The listing builds one solid part. Answer for the finished solid, in the listing's coordinates (mm). Give positions to 0.01 mm unless a question says otherwise; leave off trailing zeros. Order: outer loops, then holes, each group sorted by start corner. A loop starts at its lowest first (then second) coordinate and runs counter-clockwise, first axis right, second up. Notation, with made-up numbers: (82.25, 40.25) -> (115.25, 40.25) arc R21 cw to (115.25, 48.25) -> close; hole circle Ø9 at (-21, 4.25). An arc over 180 degrees is marked (long way). Answer as a JSON object with one key per item and string values. Group by question number.
```python
from build123d import *

# Parameters (mm, degrees)
SKETCH2_R               = 4.575
BOSS_EXTRUDE1_DEPTH     = 31.5
CUT_EXTRUDE1_DEPTH      = 33.15760019
CUT_EXTRUDE1_DEPTH_BACK = 33.15760019
SKETCH1_R               = 31
CUT_EXTRUDE2_DEPTH      = 7.524256813
CUT_EXTRUDE2_DEPTH_BACK = 7.524256813
SKETCH3_R               = 2.05


with BuildPart() as part:
    # Sketch2 → Boss-Extrude1 (new body)
    with BuildSketch(Plane(origin=(0, 0, 0), x_dir=(-1, 0, 0), z_dir=(0, 1, 0))):
        with Locations(Location((0, 0, 0), (0, 0, 90))):
            Circle(SKETCH2_R)
    extrude(amount=BOSS_EXTRUDE1_DEPTH)

    # Sketch1 → Cut-Extrude1 (cut, two sides: drawn at the far end of the back side and taken through both)
    with BuildSketch(Plane(origin=(0, 0, 0), x_dir=(0, 1, 0), z_dir=(0, 0, 1)).offset(-CUT_EXTRUDE1_DEPTH_BACK)):
        Circle(SKETCH1_R)
    extrude(amount=CUT_EXTRUDE1_DEPTH + CUT_EXTRUDE1_DEPTH_BACK, mode=Mode.SUBTRACT)

    # Sketch3 → Cut-Extrude2 (cut, two sides: drawn at the far end of the back side and taken through both)
    with BuildSketch(Plane(origin=(0, 31.5, 0), x_dir=(-1, 0, 0), z_dir=(0, 1, 0)).offset(-CUT_EXTRUDE2_DEPTH_BACK)):
        with Locations(Location((0, 0, 0), (0, 0, 90))):
            Circle(SKETCH3_R)
    extrude(amount=CUT_EXTRUDE2_DEPTH + CUT_EXTRUDE2_DEPTH_BACK, mode=Mode.SUBTRACT)


solid = part.part
```
(1) Flat-ended cylindrical pins translate along their axes: pin 1 Ø2 at (x, z) = (2, 3) entering from -Y; pin 2 Ø2 at (x, z) = (-2.5, -2) entering from -Y. Find the tip coordinate at first contact, or state that the pin passes through.
(2) Find the intervals of material crossed by line 1 along X through (y, z) = (31.25, 0) (3 decimals); line 2 along Z through (x, y) = (-0.5, 31.1), in increasing order. Write a range as [from, to].
(3) A cutting plane is placed at B-B (z = 0). Determine the outline of the cut face in (x, y) (3 decimals).
(4) A cutting plane is placed at C-C (y = 31.3). Determine the outline of the cut face in (x, z) (3 decimals), and give its area (3 significant figures).
(5) A cutting plane is placed at A-A (x = 0). Determine the outline of the cut face in (y, z) (3 decimals).
(6) For a pull along X with two mould halves and no side action, classify faces 1 (the cylindrical face through (1.08, 30.98, 1.97)), 2 (the cylindrical face through (-0.79, 31.21, 1.89)), 3 (the cylindrical face through (1.374, 31.168, 4.364)), 4 (the flat face through (-2, 31.5, 1)) as +X half, -X half, draft (parallel to the pull), parting line (faces both ways), or undercut.
(7) A cutting plane is placed at D-D (z = 3). Determine the outline of the cut face in (x, y).
Check sheet entries:
{
 "1": {"pin 1": "stops at y = 30.85", "pin 2": "stops at y = 30.8"},
 "2": {"line 1": "x = [-4.575, -2.05], [2.05, 4.575]", "line 2": "z = [-4.55, -1.99], [1.99, 4.55]"},
 "3": {"outline": "(-4.575, 30.661) arc R31 cw to (-2.05, 30.932) -> (-2.05, 31.5) -> (-4.575, 31.5) -> close; (2.05, 30.932) arc R31 cw to (4.575, 30.661) -> (4.575, 31.5) -> (2.05, 31.5) -> close"},
 "4": {"outline": "circle Ø9.15 at (0, 0); hole circle Ø4.1 at (0, 0)", "area": "52.6 mm2"},
 "5": {"outline": "(31, -4.575) -> (31.5, -4.575) -> (31.5, -2.05) -> (31, -2.05) -> close; (31, 2.05) -> (31.5, 2.05) -> (31.5, 4.575) -> (31, 4.575) -> close"},
 "6": {"face 1": "undercut", "face 2": "undercut", "face 3": "parting line", "face 4": "draft"},
 "7": {"outline": "(-3.45, 30.81) arc R31 cw to (3.45, 30.81) -> (3.45, 31.5) -> (-3.45, 31.5) -> close"}
}
